```python
from build123d import *

# Parameters (mm, degrees)
F0_W     = 9.525
F0_H     = 50.8
F2_DEPTH = 38.1
F3_DEPTH = 19.05
F5_DEPTH = 19.05
F7_DEPTH = 19.05
F8_R     = 5.55625
F9_DEPTH = 31.75


with BuildPart() as f1:
    # F0 (on Front) → F1 (revolve)
    with BuildSketch(Plane.XZ):
        with Locations((4.7625, 25.4)):
            Rectangle(F0_W, F0_H)
        Polygon((0, 101.6), (0, 50.8), (9.525, 50.8), (9.525, 0), (15.875, 0), (12.0523, 25.8093433608), (12.0523, 101.6), align=None)
        Polygon((38.1, -31.4561230436), (0, -24.7380650786), (0, -28.3439140145), (38.1, -31.6772320948), align=None)
        Polygon((38.1, -31.6772320948), (0, -28.3439140145), (0, -44.081942035), (38.1, -50.8), align=None)
        Polygon((38.1, -50.8), (0, -44.081942035), (0, -47.4666819197), align=None)
        Polygon((38.1, -50.8), (0, -47.4666819197), (0, -50.8), align=None)
        Polygon((9.525, 0), (0, 0), (0, -24.7380650786), (38.1, -31.4561230436), (38.1, -9.5908048664), (26.9875, -3.175), (15.875, -3.175), (15.875, 0), align=None)
    revolve(axis=Axis((0, 0, -25.4), (0, 0, -1)))

    # F0 (on Front) → F2 (cut, symmetric)
    with BuildSketch(Plane.XZ):
        Polygon((0, -50.8), (0, -47.4666819197), (-38.1, -44.1333638393), (-38.1, -50.8), align=None)
        Polygon((38.1, -50.8), (0, -47.4666819197), (0, -50.8), align=None)
    extrude(amount=F2_DEPTH, both=True, mode=Mode.SUBTRACT)

    # F0 (on Front) → F3 (cut)
    with BuildSketch(Plane.XZ):
        Polygon((38.1, -31.6772320948), (0, -28.3439140145), (0, -44.081942035), (38.1, -50.8), align=None)
        Polygon((0, -44.081942035), (0, -28.3439140145), (-35.954874027, -25.1982701386), (-36.9244921743, -30.6972479093), (-37.5167449121, -37.4667276786), align=None)
        Polygon((0, -47.4666819197), (0, -44.081942035), (-37.5167449121, -37.4667276786), (-38.1, -44.1333638393), align=None)
        Polygon((38.1, -50.8), (0, -44.081942035), (0, -47.4666819197), align=None)
        Polygon((-36.9244921743, -30.6972479093), (-35.954874027, -25.1982701386), (-36.4396831007, -25.1558548407), align=None)
        Polygon((-38.1, -37.36388407), (-36.9244921743, -30.6972479093), (-36.4396831007, -25.1558548407), (-38.1, -25.0105959341), align=None)
        Polygon((-38.1, -37.36388407), (-37.5167449121, -37.4667276786), (-36.9244921743, -30.6972479093), align=None)
        Polygon((-38.1, -44.1333638393), (-37.5167449121, -37.4667276786), (-38.1, -37.36388407), align=None)
    extrude(amount=-F3_DEPTH, mode=Mode.SUBTRACT)

    # F4 (on face) → F5 (cut)
    with BuildSketch(Plane(origin=(-4.1212514076, 0, -47.106119142), x_dir=(0.9961946981, 0, -0.0871557427), z_dir=(-0.0871557427, 0, -0.9961946981))):
        with BuildLine():
            Line((-28.9846116747, 19.05), (4.5792120209, 19.05))
            Line((4.5792120209, 19.05), (37.2585995116, 19.05))
            add(Edge.make_bspline(
                [(4.1369939185, 38.1), (26.2180643139, 38.1), (37.2585995116, 19.05)],
                knots=[1.5707963268, 1.5707963268, 1.5707963268, 2.6058232788, 2.6058232788, 2.6058232788], degree=2, weights=[1, 0.8070072037, 0.8683475024]))
            add(Edge.make_bspline(
                [(-28.9846116747, 19.05), (-17.944076477, 38.1), (4.1369939185, 38.1)],
                knots=[0.5357693748, 0.5357693748, 0.5357693748, 1.5707963268, 1.5707963268, 1.5707963268], degree=2, weights=[0.8683475024, 0.8070072037, 1]))
        make_face()
        with BuildLine():
            Line((-34.1085418919, 19.05), (-28.9846116747, 19.05))
            add(Edge.make_bspline(
                [(-28.9846116747, 19.05), (-17.944076477, 38.1), (4.1369939185, 38.1)],
                knots=[0.5357693748, 0.5357693748, 0.5357693748, 1.5707963268, 1.5707963268, 1.5707963268], degree=2, weights=[0.8683475024, 0.8070072037, 1]))
            Line((4.1369939185, 38.1), (-34.1085418919, 38.1365224015))
            Line((-34.1085418919, 38.1365224015), (-34.1085418919, 19.05))
        make_face()
    extrude(amount=-F5_DEPTH, mode=Mode.SUBTRACT)

    # F6 (on face) → F7 (cut)
    with BuildSketch(Plane.XZ.offset(19.05)):
        with BuildLine():
            Line((3.1629181664, -38.1820174503), (-3.1629181664, -37.6285784838))
            ThreePointArc((-3.1629181664, -37.6285784838), (-0.2767194832, -41.0682161335), (3.1629181664, -38.1820174503))
        make_face()
        with BuildLine():
            ThreePointArc((3.175, -37.9052979671), (0.1384915549, -34.7333198635), (-3.1629181664, -37.6285784838))
            Line((-3.1629181664, -37.6285784838), (3.1629181664, -38.1820174503))
            ThreePointArc((3.1629181664, -38.1820174503), (3.1719781035, -38.0437895219), (3.175, -37.9052979671))
        make_face()
        with BuildLine():
            ThreePointArc((-22.225, -35.6830859135), (-25.2615084451, -32.51110781), (-28.5629181664, -35.4063664303))
            Line((-28.5629181664, -35.4063664303), (-22.2370818336, -35.9598053967))
            ThreePointArc((-22.2370818336, -35.9598053967), (-22.2280218965, -35.8215774684), (-22.225, -35.6830859135))
        make_face()
        with BuildLine():
            Line((-22.2370818336, -35.9598053967), (-28.5629181664, -35.4063664303))
            ThreePointArc((-28.5629181664, -35.4063664303), (-25.6767194832, -38.8460040799), (-22.2370818336, -35.9598053967))
        make_face()
        with BuildLine():
            ThreePointArc((22.2370818336, -39.8507905374), (25.1232805168, -43.2904281871), (28.5629181664, -40.4042295038))
            Line((28.5629181664, -40.4042295038), (22.2370818336, -39.8507905374))
        make_face()
        with BuildLine():
            Line((22.2370818336, -39.8507905374), (28.5629181664, -40.4042295038))
            ThreePointArc((28.5629181664, -40.4042295038), (28.5719781035, -40.2660015755), (28.575, -40.1275100206))
            ThreePointArc((28.575, -40.1275100206), (25.5384915549, -36.9555319171), (22.2370818336, -39.8507905374))
        make_face()
    extrude(amount=-F7_DEPTH, mode=Mode.SUBTRACT)

    # F8 (on face) → F9 (cut)
    with BuildSketch(Plane.XY.offset(101.6)):
        Circle(F8_R)
    extrude(amount=-F9_DEPTH, mode=Mode.SUBTRACT)


solid = f1.part
```
Geometry check sheet. Reference: the model listing, model coordinates, mm. A direction names the side the tool comes from. Coordinates: 2 decimals unless noted, no trailing zeros. Order: outer loops, then holes, each group sorted by start corner. A loop starts at its lowest first (then second) coordinate and runs counter-clockwise, first axis right, second up. Notation, with made-up numbers: (-25.5, 1.5) - (-8.5, 1.5) arc R24 ccw to (-8.5, 38.5) - close; hole circle Ø1 at (74.5, 6). An arc over 180 degrees is marked (long way). Answer in a Markdown table with one row per item. Add a question column.
1. Material ranges on L1, parallel to Y at x = 0, z = 86; L2, parallel to Y at x = -28, z = -40.5; L3, parallel to Z at x = -25, y = -7 (3 decimals), recorded low to high. Write a range as [from, to].
2. Access from +Z, -Z, +X, -X, +Y, -Y to the whole of each face (thin tool, end or side, straight path). Record for faces 1 (the face through (12, 12, -3.175)), 2 (the face through (5, 3, 101.6)), 3 (the face through (-8.259, 37.194, -25.328)), 4 (the face through (-1, 0, -43)), 5 (the face through (-1, -19.05, -42)).
3. Draft check along X on faces 6 (the face through (0, 19.05, -38)), 7 (the face through (-3.583, -27.293, -3.487)), 8 (the face through (-0.5, -26.6, -28.3)), 9 (the face through (5.3, 1.67, 85.95)). Enter one of: +X half, -X half, draft (parallel to the pull), parting line (faces both ways), or undercut.
4. Gauge pin test, flat ends, axial feed: pin 1 Ø3 at (x, y) = (2.5, 26) entering from +Z (3 decimals); pin 2 Ø5.5 at (x, y) = (2.5, 1) entering from +Z; pin 3 Ø2 at (x, z) = (7, -10) entering from +Y. Record the tip position at first contact, or that the pin passes through.
5. Section check B-B (z = 5). Enter the section's corners in (x, y).
6. Section check A-A (z = 47). Enter the section's corners in (x, y).
Data:
| question | item | result |
|---|---|---|
| 1 | L1 | y = [-12.05, -5.56], [5.56, 12.05] |
| 1 | L2 | y = [-19.05, 0], [19.05, 25.84] |
| 1 | L3 | z = [-45.279, -38.833], [-32.533, -3.175] |
| 2 | face 1 | +Z |
| 2 | face 2 | +Z, +X, -X, +Y, -Y |
| 2 | face 3 | +Z, -Z |
| 2 | face 4 | -Z, -X |
| 2 | face 5 | -Z, -X, -Y |
| 3 | face 6 | draft |
| 3 | face 7 | parting line |
| 3 | face 8 | -X half |
| 3 | face 9 | undercut |
| 4 | pin 1 | stops at z = -3.175 |
| 4 | pin 2 | stops at z = 69.85 |
| 4 | pin 3 | stops at y = 37.62 |
| 5 | outline | circle Ø30.27 at (0, 0) |
| 6 | outline | circle Ø24.1 at (0, 0) |
